The model under review builds one solid part; all positions refer to its coordinate system, in mm. A direction names the side the tool comes from. Round coordinates to 2 decimals unless told otherwise and drop trailing zeros. Order: outer loops, then holes, each group sorted by start corner. A loop starts at its lowest first (then second) coordinate and runs counter-clockwise, first axis right, second up. Notation, with made-up numbers: M 79.25,13.25 L 108.25,13.25 A6 ccw 108.25,22.25 Z; hole C -9,-9.75 d7. An arc over 180 degrees is marked long. Use a Markdown table: item, result. Add a question column.
1. The part is to be moulded in two halves that separate along X. For faces 5 (the flat face through (6, 4, -49)), 6 (the flat face through (3, 7, -39)), 7 (the flat face through (0, 4, -49)), 8 (the flat face through (0.3, 4.1, 0)), say which applies: +X half, -X half, draft (parallel to the pull), parting line (faces both ways), or undercut.
2. To check wall thickness, follow probe 1 along Y at (x, z) = (2.5, -76.5); probe 2 along X at (y, z) = (7.75, -20); probe 3 along X at (y, z) = (2.75, -57). State the ranges of each line that lie inside material, in increasing order.
3. For faces 1 (the flat face through (3, 4, -80)), 2 (the cylindrical face through (2.63, 7.49, -19.29)), 3 (the cylindrical face through (3.577, 2.891, -94.93)), 4 (the flat face through (3, 8, -49)), list the 3-axis set-ups (+Z, -Z, +X, -X, +Y, -Y) from which the entire face can be reached by the end or side of a thin tool; tool diameter is ignored.
4. Consider section A-A on z = -16. State the section outline as (x, y) points.
5. Insertion check: P1, Ø1, axis at x = 2, y = 1, coming from the +Z side; P2, Ø1.4, axis at x = 3, z = -20, coming from the +Y side; P3, Ø2, axis at x = 3, y = 4, coming from the +Z side. Each pin has a flat end and moves straight along its axis. Give the tip position at first contact, or say it passes through.
from build123d import *

# Parameters (mm, degrees)
ESQUISSE1_W             = 6
ESQUISSE1_H             = 8
BOSS_EXTRU_1_DEPTH      = 100
ESQUISSE2_W             = 4
ESQUISSE2_H             = 6
ENL_V_MAT_EXTRU_1_DEPTH = 80
TROU_TARAUD_M21_D       = 1.6
TROU_TARAUD_M21_DEPTH   = 4
TROU_TARAUD_M21_TIP     = 0.480688495
TROU_TARAUD_M31_D       = 2.5
TROU_TARAUD_M31_DEPTH   = 10
TROU_TARAUD_M31_TIP     = 0.751075774


with BuildPart() as part:
    # Esquisse1 → Boss.-Extru.1 (new body)
    with BuildSketch(Plane.XY):
        with Locations((3, 4)):
            Rectangle(ESQUISSE1_W, ESQUISSE1_H)
    extrude(amount=-BOSS_EXTRU_1_DEPTH)

    # Esquisse2 → Enlèv. mat.-Extru.1 (cut)
    with BuildSketch(Plane.XY):
        with Locations((3, 4)):
            Rectangle(ESQUISSE2_W, ESQUISSE2_H)
    extrude(amount=-ENL_V_MAT_EXTRU_1_DEPTH, mode=Mode.SUBTRACT)

    # Trou taraudé M21
    with Locations(Plane(origin=(0, 8, 0), x_dir=(1, 0, 0), z_dir=(0, 1, 0))):
        with Locations((3, 20)):
            Hole(TROU_TARAUD_M21_D / 2, depth=TROU_TARAUD_M21_DEPTH)
            with Locations((0, 0, -(TROU_TARAUD_M21_DEPTH + TROU_TARAUD_M21_TIP / 2))):  # 118° drill point
                Cone(0, TROU_TARAUD_M21_D / 2, TROU_TARAUD_M21_TIP, mode=Mode.SUBTRACT)

    # Trou taraudé M31
    with Locations(Plane(origin=(0, 0, -100), x_dir=(-1, 0, 0), z_dir=(0, 0, -1))):
        with Locations((-3, 4)):
            Hole(TROU_TARAUD_M31_D / 2, depth=TROU_TARAUD_M31_DEPTH)
            with Locations((0, 0, -(TROU_TARAUD_M31_DEPTH + TROU_TARAUD_M31_TIP / 2))):  # 118° drill point
                Cone(0, TROU_TARAUD_M31_D / 2, TROU_TARAUD_M31_TIP, mode=Mode.SUBTRACT)


solid = part.part
Answer block:
| question | item | result |
|---|---|---|
| 1 | face 5 | +X half |
| 1 | face 6 | undercut |
| 1 | face 7 | -X half |
| 1 | face 8 | draft |
| 2 | probe 1 | 0 to 1, 7 to 8 |
| 2 | probe 2 | 0 to 2.2, 3.8 to 6 |
| 2 | probe 3 | 0 to 1, 5 to 6 |
| 3 | face 1 | +Z |
| 3 | face 2 | +Y |
| 3 | face 3 | -Z |
| 3 | face 4 | +Z, -Z, +X, -X, +Y |
| 4 | outline | M 0,0 L 6,0 L 6,8 L 0,8 Z; hole M 1,1 L 5,1 L 5,7 L 1,7 Z |
| 5 | P1 | z = 0 |
| 5 | P2 | y = 1 |
| 5 | P3 | z = -80 |
